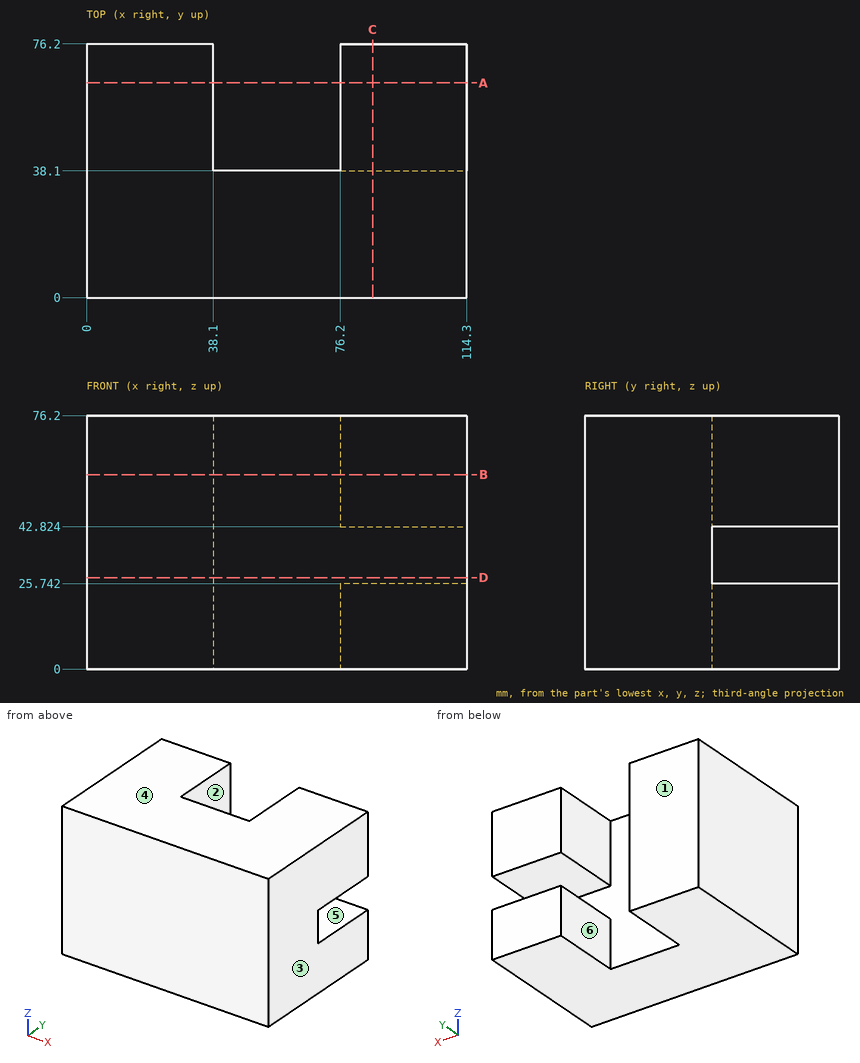
Print and shaded views of the part. All mm, measured from the part's lowest x, y and z. A direction names the side the tool comes from. Round coordinates to 2 decimals unless told otherwise and drop trailing zeros. Write each loop counter-clockwise with the first axis right and the second up, starting at its lowest first coordinate (ties: lowest second). Pieces come first, ordered by that corner, then holes.
(1) 3-axis set-ups, long thin cutter, end or side, ignore diameter. For the marked faces 4, 5 and 6: which of +Z, -Z, +X, -X, +Y, -Y reach the whole face in a straight line?
(2) Slice it at B-B, the plane z = 58.5. Write the cut outline in (x, y), and give its area (3 significant figures).
(3) Drop a flat-ended pin along its axis: P1, Ø11.5, axis at y = 48.5, z = 35.5, coming from the +X side. Give the stop position or say it passes through.
(4) Slice it at C-C, the plane x = 86. Write the cut outline in (y, z), and give its area (3 significant figures).
(5) Slice it at D-D, the plane z = 27.5. Write the cut outline in (x, y), and give its area (3 significant figures).
(6) Slice it at A-A, the plane y = 64.5. Write the cut outline in (x, z).
(7) Mould opens along X. For the marked faces 1, 2 and 3 say: pulls with the +X half, pulls with the -X half, needs draft (parallel to the pull), parting line crosses it, or undercut.
(8) Probe line 1 along X through (y, z) = (51, 18); line 2 along Z through (x, y) = (100, 61); line 3 along Y through (x, z) = (43.5, 26). List the from-to ranges inside material, lowest first.
From the geometry:
1. face 4: +Z, +X, -X, +Y, -Y
1. face 5: +X, +Y
1. face 6: +Z, -Z, +Y
2. outline: (0, 0) - (114.3, 0) - (114.3, 76.2) - (76.2, 76.2) - (76.2, 38.1) - (38.1, 38.1) - (38.1, 76.2) - (0, 76.2) - close
2. area: 7,260 mm2
3. P1: stops at x = 38.1
4. outline: (0, 0) - (76.2, 0) - (76.2, 25.74) - (38.1, 25.74) - (38.1, 42.82) - (76.2, 42.82) - (76.2, 76.2) - (0, 76.2) - close
4. area: 5,160 mm2
5. outline: (0, 0) - (114.3, 0) - (114.3, 38.1) - (38.1, 38.1) - (38.1, 76.2) - (0, 76.2) - close
5. area: 5,810 mm2
6. outline: (0, 0) - (38.1, 0) - (38.1, 76.2) - (0, 76.2) - close; (76.2, 0) - (114.3, 0) - (114.3, 25.74) - (76.2, 25.74) - close; (76.2, 42.82) - (114.3, 42.82) - (114.3, 76.2) - (76.2, 76.2) - close
7. face 1: needs draft
7. face 2: undercut
7. face 3: pulls with the +X half
8. line 1: x = 0 to 38.1, 76.2 to 114.3
8. line 2: z = 0 to 25.74, 42.82 to 76.2
8. line 3: y = 0 to 38.1
